Source: CAD feature listing. Evaluate the final solid. Frame: model axes, mm. Coordinates: 2 decimals unless noted, no trailing zeros. Loops run counter-clockwise (first coordinate to the right, second up) from the corner with the lowest first, then second, coordinate; pieces in that order, holes last. Notation, with made-up numbers: M 28.25,-32 L 74.25,-32 A30 ccw 74.25,1 Z; hole C -24,-26.75 d2. An arc over 180 degrees is marked long. One line per question, with ' | ' between items. Start each with the question number.
1. Ray query, probe 1 along X at (y, z) = (3.5, -65); probe 2 along Z at (x, y) = (78, 8.5); probe 3 along Z at (x, y) = (32.1, 3.25). Return the intervals inside material, ascending.
2. Section query C-C, the plane x = 82.1. Output: boundary loops of the cut face in (y, z).
3. Section query A-A, the plane x = 32.1. Output: boundary loops of the cut face in (y, z), and give its area (3 significant figures).
4. Section query D-D, the plane x = 59. Output: boundary loops of the cut face in (y, z), and give its area (3 significant figures).
5. Mould query, pull axis X, two halves, no side actions, for faces 1 (the cylindrical face through (65.821, 4.93, -110.222)), 2 (the flat face through (7, 5, -127)), 3 (the cylindrical face through (17.69, 4.93, -116.2)), 4 (the flat face through (0, 5, -63)). Classes: pulls with the +X half, pulls with the -X half, needs draft (parallel to the pull), parting line crosses it, or undercut.
6. Section query B-B, the plane y = 7. Output: boundary loops of the cut face in (x, z), and give its area (3 significant figures).
7. Pin query (flat end, axial travel): P1, Ø8, axis at x = 32.1, z = -65, coming from the -Y side. Return the tip coordinate at first contact, or that it passes through.
```python
from build123d import *

# Parameters (mm, degrees)
BOSS_EXTRUDE1_DEPTH     = 10
SKETCH2_R               = 5
CUT_EXTRUDE4_DEPTH      = 11
CUT_EXTRUDE4_DEPTH_BACK = 1


with BuildPart() as part:
    # Sketch1 → Boss-Extrude1 (new body)
    with BuildSketch(Plane(origin=(0, 0, 0), x_dir=(1, 0, 0), z_dir=(0, 1, 0))):
        with BuildLine():
            Line((0, 0), (0, 127))
            Line((0, 127), (15, 127))
            ThreePointArc((15, 127), (66.440280909, 109.758742946), (97.1, 65))
            Line((97.1, 65), (97.1, 0))
            Line((97.1, 0), (0, 0))
        make_face()
    extrude(amount=BOSS_EXTRUDE1_DEPTH)

    # Sketch2 → Cut-Extrude4 (cut, two sides)
    with BuildSketch(Plane(origin=(0, 0, 0), x_dir=(1, 0, 0), z_dir=(0, 1, 0))) as cut_extrude4_sk:
        with Locations((14.998992834, 111.984631039)):
            Circle(SKETCH2_R)
        with Locations((82.1, 65)):
            Circle(SKETCH2_R)
        with Locations((32.1, 65)):
            Circle(SKETCH2_R)
    extrude(amount=CUT_EXTRUDE4_DEPTH, mode=Mode.SUBTRACT)
    extrude(cut_extrude4_sk.sketch, amount=-CUT_EXTRUDE4_DEPTH_BACK, mode=Mode.SUBTRACT)


solid = part.part
```
Taken from the geometry:
1) probe 1: 0 to 27.1, 37.1 to 77.1, 87.1 to 97.1 | probe 2: -99.24 to -67.86, -62.14 to 0 | probe 3: -125.27 to -70, -60 to 0
2) outline: M 0,-94.4 L 10,-94.4 L 10,-70 L 0,-70 Z; M 0,-60 L 10,-60 L 10,0 L 0,0 Z
3) outline: M 0,-125.27 L 10,-125.27 L 10,-70 L 0,-70 Z; M 0,-60 L 10,-60 L 10,0 L 0,0 Z | area: 1,150 mm^2
4) outline: M 0,-114.79 L 10,-114.79 L 10,0 L 0,0 Z | area: 1,150 mm^2
5) face 1: pulls with the +X half | face 2: needs draft | face 3: undercut | face 4: pulls with the -X half
6) outline: M 0,-127 L 15,-127 A85.36 ccw 97.1,-65 L 97.1,0 L 0,0 Z; hole C 15,-111.98 d10; hole C 32.1,-65 d10; hole C 82.1,-65 d10 | area: 10,800 mm^2
7) P1: through
